from build123d import *

# Parameters (mm, degrees)
SKETCH1_W           = 142.755639788
SKETCH1_H           = 271.365530146
BOSS_EXTRUDE1_DEPTH = 12.7
HOLE1_D             = 3.175
HOLE1_DEPTH         = 31.75
HOLE1_CSINK_D       = 10.16
HOLE1_CSINK_ANGLE   = 82
HOLE1_TIP           = 0.953866233


with BuildPart() as part:
    # Sketch1 → Boss-Extrude1 (new body)
    with BuildSketch(Plane.XY):
        with Locations((-163.375147287, -52.841023691)):
            Rectangle(SKETCH1_W, SKETCH1_H)
    extrude(amount=BOSS_EXTRUDE1_DEPTH)

    # Hole1
    with Locations(Plane(origin=(181.039434513, -52.974999997, 0), x_dir=(0, -1, 0), z_dir=(0, 0, -1))):
        with Locations((129.198788767, 384.042401694), (-129.466741379, 384.042401694), (-129.466741379, 304.786761906), (-110.416741379, 409.442401694), (-0.133976306, 409.442401694), (110.148788767, 409.442401694), (129.198788767, 304.786761906)):
            CounterSinkHole(HOLE1_D / 2, HOLE1_CSINK_D / 2, depth=HOLE1_DEPTH, counter_sink_angle=HOLE1_CSINK_ANGLE)
            with Locations((0, 0, -(HOLE1_DEPTH + HOLE1_TIP / 2))):  # 118° drill point
                Cone(0, HOLE1_D / 2, HOLE1_TIP, mode=Mode.SUBTRACT)


solid = part.part
Work out the finished part from the listing and answer in its coordinate system (mm). Give positions to 0.01 mm unless a question says otherwise; leave off trailing zeros. Answer as a JSON object with one key per item and string values. Group by question number.
1. The mould has two halves that part along Y. Classify faces 1 (the flat face through (-164, -188.524, 6)), 2 (the flat face through (-164, 82.842, 6)), 3 (the conical face through (-228.931, -161.448, 3.823)): released by +Y, released by -Y, zero draft, split by the parting line, or undercut.
2. Flat-ended cylindrical pins translate along their axes: pin 1 Ø4 at (x, y) = (-203, 76.49) entering from -Z; pin 2 Ø3.5 at (x, y) = (-228.4, -52.84) entering from -Z. Find the tip coordinate at first contact, or state that the pin passes through.
3. Consider line 1 along Y through (x, z) = (-125, 3); line 2 along X through (y, z) = (-164, 11). Determine where each line is inside the solid, lowest interval first. Write a range as [from, to].
Result sheet:
{
 "1": {"face 1": "released by -Y", "face 2": "released by +Y", "face 3": "undercut"},
 "2": {"pin 1": "stops at z = 3.54", "pin 2": "stops at z = 3.83"},
 "3": {"line 1": "y = [-188.52, -184.31], [-180.04, 74.36], [78.62, 82.84]", "line 2": "x = [-234.75, -229.73], [-227.08, -92]"}
}
